Verification items for the finished model (mm, model axes). Coordinates: 2 decimals unless noted, no trailing zeros. Order: outer loops, then holes, each group sorted by start corner. A loop starts at its lowest first (then second) coordinate and runs counter-clockwise, first axis right, second up. Notation, with made-up numbers: (-32.75, -23) -> (-0.75, -23) arc R28 cw to (-0.75, 10) -> close; hole circle Ø1 at (18, 14). An arc over 180 degrees is marked (long way). Use CSV: the item, a comma, the result in double quotes. Start each with the question number.
1) Scan lines: line 1 along X through (y, z) = (-12.5, -25); line 2 along Z through (x, y) = (-63, -14.5); line 3 along Z through (x, y) = (-51.5, -1.5). Record each from-to range of solid material in increasing order.
2) Sectioned sample at A-A on x = -56. Record the boundary of the cut face in (y, z), then the cut area to 3 significant figures.
3) Go/stop test with flat-tipped pins: pin 1 (6 mm diameter, centred on x = -45.5, y = -15.5, fed in from +Z); pin 2 (1 mm diameter, centred on y = -16, z = -19.5, fed in from +X); pin 3 (6 mm diameter, centred on x = -57, y = -5, fed in from +Z). Record where each tip stops, or that it passes through.
from build123d import *

# Parameters (mm, degrees)
F1_DEPTH = 25.4


with BuildPart() as f1:
    # F0 (on Front) → F1 (new body)
    with BuildSketch(Plane.XZ):
        with BuildLine():
            add(Edge.make_bspline(
                [(-18.2338618332, 35.049978312), (-16.2634742331, 33.5219960414), (-14.3632449685, 32.0948882514), (-12.5260129681, 30.7620231507)],
                knots=[0, 0, 0, 0, 0.065741729, 0.065741729, 0.065741729, 0.065741729], degree=3))
            ThreePointArc((-18.2338618332, 35.049978312), (-71.2893804123, 4.6016135845), (-17.4403864611, -24.4203921477))
            add(Edge.make_bspline(
                [(-17.4403864611, -24.4203921477), (-17.179402441, -24.2472786453), (-16.9196286438, -24.0762946974), (-16.6610557268, -23.9074107575)],
                knots=[0, 0, 0, 0, 0.0086559059, 0.0086559059, 0.0086559059, 0.0086559059], degree=3))
            ThreePointArc((-16.6610557268, -23.9074107575), (-5.3724339888, -11.3311344475), (-1.2924953236, 5.0685547891))
            ThreePointArc((-1.2924953236, 5.0685547891), (-4.2236094492, 19.0894876674), (-12.5260129681, 30.7620231507))
        make_face()
        with BuildLine():
            ThreePointArc((-12.5260129681, 30.7620231507), (-15.2703232487, 33.0519120082), (-18.2338618332, 35.049978312))
            add(Edge.make_bspline(
                [(-18.2338618332, 35.049978312), (-16.2634742331, 33.5219960414), (-14.3632449685, 32.0948882514), (-12.5260129681, 30.7620231507)],
                knots=[0, 0, 0, 0, 0.065741729, 0.065741729, 0.065741729, 0.065741729], degree=3))
        make_face()
        with BuildLine():
            add(Edge.make_bspline(
                [(-17.4403864611, -24.4203921477), (-17.179402441, -24.2472786453), (-16.9196286438, -24.0762946974), (-16.6610557268, -23.9074107575)],
                knots=[0, 0, 0, 0, 0.0086559059, 0.0086559059, 0.0086559059, 0.0086559059], degree=3))
            ThreePointArc((-17.4403864611, -24.4203921477), (-17.0490116738, -24.1664984351), (-16.6610557268, -23.9074107575))
        make_face()
        with BuildLine():
            add(Edge.make_bspline(
                [(-12.5260129681, 30.7620231507), (2.638402042, 19.7606256484), (20.1903372376, 12.3655817594), (38.1732838608, 11.9589753306), (38.6908322584, 12.4428219154), (38.7721241334, 12.5086976901)],
                knots=[0.065741729, 0.065741729, 0.065741729, 0.065741729, 0.6083704565, 0.9417253051, 1, 1, 1, 1], degree=3))
            ThreePointArc((-12.5260129681, 30.7620231507), (-4.2236094492, 19.0894876674), (-1.2924953236, 5.0685547891))
            ThreePointArc((-1.2924953236, 5.0685547891), (-5.3724339888, -11.3311344475), (-16.6610557268, -23.9074107575))
            add(Edge.make_bspline(
                [(-16.6610557268, -23.9074107575), (2.0260763524, -11.7021244239), (14.4410223527, -10.4651605814), (24.1103417725, -9.0437679707)],
                knots=[0.0086559059, 0.0086559059, 0.0086559059, 0.0086559059, 0.6342204815, 0.6342204815, 0.6342204815, 0.6342204815], degree=3))
            add(Edge.make_bspline(
                [(24.1103417725, -9.0437679707), (29.6806384765, -8.2249328253), (34.3397507009, -7.3448917488), (38.5815591641, -7.5473355981)],
                knots=[0.6342204815, 0.6342204815, 0.6342204815, 0.6342204815, 0.9945954099, 0.9945954099, 0.9945954099, 0.9945954099], degree=3))
            add(Edge.make_bspline(
                [(38.5815591641, -7.5473355981), (38.6450808205, -0.6026015768), (38.708602477, 5.5213805001), (38.7721241334, 12.5086976901)],
                knots=[0.5076766633, 0.5076766633, 0.5076766633, 0.5076766633, 20.5853675478, 20.5853675478, 20.5853675478, 20.5853675478], degree=3))
        make_face()
    extrude(amount=F1_DEPTH)


solid = f1.part
Answers follow:
1,line 1,"x = -54.21 to -18.38"
1,line 2,"z = -17.55 to 27.69"
1,line 3,"z = -26.45 to 36.59"
2,outline,"(-25.4, -23.86) -> (0, -23.86) -> (0, 33.99) -> (-25.4, 33.99) -> close"
2,area,"1,470 mm²"
3,pin 1,"stops at z = 39.51"
3,pin 2,"stops at x = -8.45"
3,pin 3,"stops at z = 35.26"
